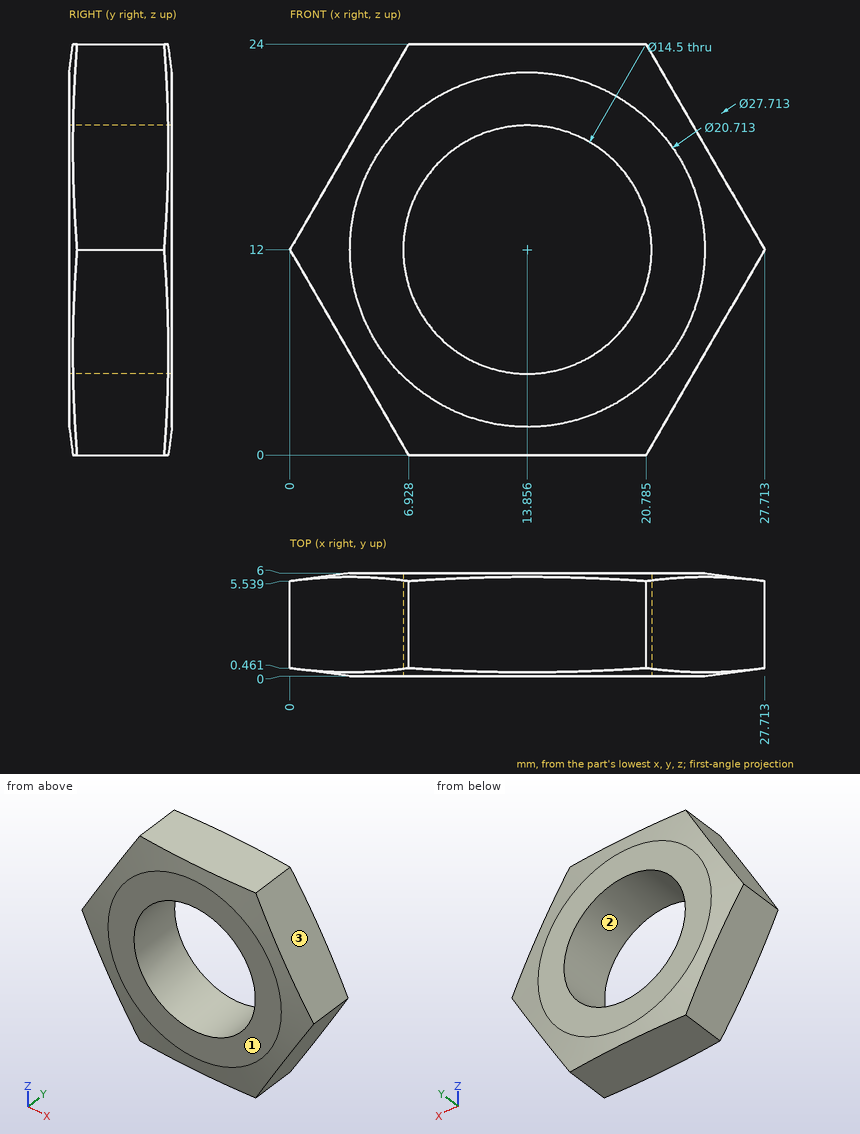
Verification items for this drawing (mm, ordinates from the low corner). Give positions to 0.01 mm unless a question says otherwise; leave off trailing zeros. Answer as a JSON object with one key per item and string values. Group by question number.
Item 1: Gauge pin test, flat end, axial feed: pin 1 (1 mm diameter, centred on x = 5.5, y = 0.5, fed in from -Z). Record the tip position at first contact, or that the pin passes through.
Item 2: Mould release check, pull along Z, two halves, no side actions. Record for the marked faces 1, 2 and 3: pulls with the +Z half, pulls with the -Z half, needs draft (parallel to the pull), parting line crosses it, or undercut.
Item 3: Material ranges on L1, parallel to Z at x = 15, y = 2; L2, parallel to Z at x = 20.5, y = 1.75 (1 decimal); L3, parallel to X at y = 1.7, z = 14.75 (1 decimal), recorded low to high.
Findings below:
{
 "1": {"pin 1": "z = 1.61"},
 "2": {"face 1": "needs draft", "face 2": "undercut", "face 3": "pulls with the +Z half"},
 "3": {"L1": "0 to 4.84, 19.16 to 24", "L2": "0 to 9.1, 14.9 to 24", "L3": "1.6 to 7.1, 20.6 to 26.1"}
}
